Job drawing, mm, ordinate dimensions from the low corner. One solid piece. Give positions to 0.01 mm unless a question says otherwise; leave off trailing zeros. Order: outer loops, then holes, each group sorted by start corner. A loop starts at its lowest first (then second) coordinate and runs counter-clockwise, first axis right, second up. Notation, with made-up numbers: (-24, -38.75) - (13, -38.75) arc R28 ccw to (13, -11.75) - close; hole circle Ø4 at (84.5, 18.25). An arc over 180 degrees is marked (long way). Write each question's results on one line, items separated by ' | '. Start each with the question number.
1) Cut at A-A on y = 1.75. List the corners of the cut face in (x, z) (1 decimal).
2) Cut at C-C on z = 13. List the corners of the cut face in (x, y).
3) Drop flat-ended pins along their axis: pin 1 Ø3 at (x, z) = (32.5, 25.5) entering from -Y; pin 2 Ø5 at (x, y) = (17, 7) entering from -Z (1 decimal); pin 3 Ø5 at (y, z) = (2, 5) entering from -X (1 decimal); pin 4 Ø4 at (y, z) = (4.5, 29) entering from +X. Give the stop position or say it passes through.
4) Cut at B-B on x = 12. List the corners of the cut face in (y, z), plus the area to 3 significant figures.
5) Drill centre lines: line 1 along X through (y, z) = (5, 4) (1 decimal); line 2 along X through (y, z) = (1, 3) (1 decimal); line 3 along Z through (x, y) = (5, 0.5). Where is each one in solid material? Low to high. Write a range as from..to.
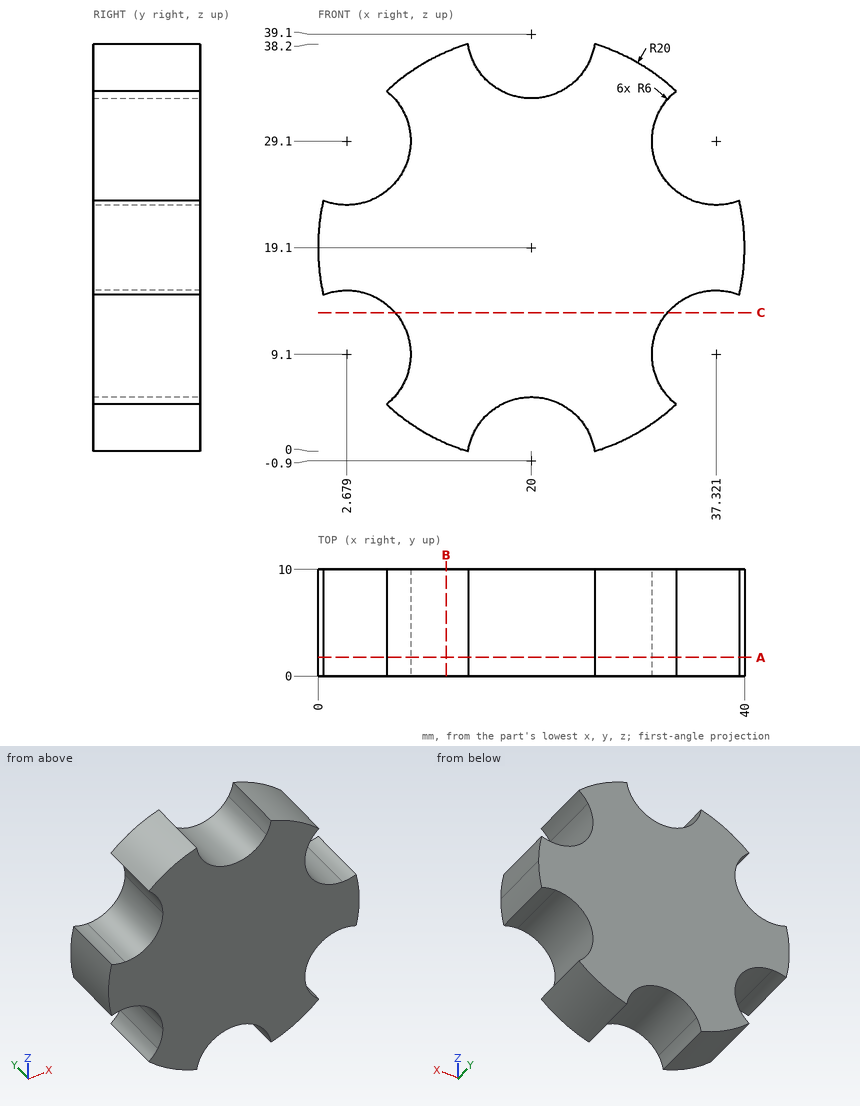
Results:
1) outline: (0.5, 14.7) arc R6 cw to (6.4, 4.4) arc R20 ccw to (14.1, 0) arc R6 cw to (25.9, 0) arc R20 ccw to (33.6, 4.4) arc R6 cw to (39.5, 14.7) arc R20 ccw to (39.5, 23.5) arc R6 cw to (33.6, 33.8) arc R20 ccw to (25.9, 38.2) arc R6 cw to (14.1, 38.2) arc R20 ccw to (6.4, 33.8) arc R6 cw to (0.5, 23.5) arc R20 ccw to start
2) outline: (7.24, 0) - (32.76, 0) - (32.76, 10) - (7.24, 10) - close
3) pin 1: y = 0 | pin 2: z = 1.5 | pin 3: x = 6.4 | pin 4: x = 31.7
4) outline: (0, 0.77) - (10, 0.77) - (10, 37.43) - (0, 37.43) - close | area: 367 mm^2
5) line 1: 6.9..16.5, 23.5..33.1 | line 2: 8.1..15.4, 24.6..31.9 | line 3: 14.63..23.57
